Input: part model. Units: mm. Frame: model coordinates. A direction names the side the tool comes from. Round coordinates to 2 decimals unless told otherwise and drop trailing zeros. Loops run counter-clockwise (first coordinate to the right, second up) from the corner with the lowest first, then second, coordinate; pieces in that order, holes last. Notation, with made-up numbers: (80.25, -7) -> (119.25, -7) arc R6 cw to (119.25, 2) -> close; hole circle Ø8 at (27, -7). An arc over 180 degrees is marked (long way). One line per question, with ' | ' between items. Start each with the question number.
Q1. Access query for faces 4 (the face through (3, -15, 7.938)), 5 (the face through (-4.336, -19.524, 2.348)), 6 (the face through (-1, -22, 0)). Directions: +Z, -Z, +X, -X, +Y, -Y. A direction counts if a zero-diameter tool reaches every point of the face in a straight line with its end or side. Return the directions, or none.
Q2. Mould query, pull axis X, two halves, no side actions, for faces 1 (the face through (-1, -22, 12.7)), 2 (the face through (3, -15, 4.762)), 3 (the face through (47.69, 15.02, 6.26)). Classes: pulls with the +X half, pulls with the -X half, needs draft (parallel to the pull), parting line crosses it, or undercut.
Q3. Cut plane D-D on y = 28. Return loops of the section in (x, z).
Q4. Cut plane C-C on z = 3.25. Return loops of the section in (x, y), and give its area (3 significant figures).
Q5. Cut plane A-A on y = 0. Return loops of the section in (x, z), and give its area (3 significant figures).
Q6. Contact query for flat-ended pins moving along their axis: P1, Ø5, axis at x = 31, z = 8, coming from the +Y side; P2, Ø5, axis at y = 5.5, z = 8.5, coming from the +X side; P3, Ø1, axis at x = -32, z = 8, coming from the -Y side; P4, Ø12, axis at x = 3.5, y = -3, coming from the +Z side. Output: stop coordinate, or through.
Q7. Material intervals for L1, parallel to Y at x = 0, z = 9.65; L2, parallel to Y at x = 0, z = 5.75; L3, parallel to X at y = 18, z = 1, sorted ascending.
from build123d import *

# Parameters (mm, degrees)
F0_R     = 50
F0_R_2   = 20
F1_DEPTH = 12.7
F3_R     = 20
F3_R_2   = 15
F4_DEPTH = 1.5875


with BuildPart() as f1:
    # F0 (on Top) → F1 (new body)
    with BuildSketch(Plane.XY):
        Circle(F0_R)
        Circle(F0_R_2, mode=Mode.SUBTRACT)
    extrude(amount=F1_DEPTH)

    # F3 (on mid) → F4 (join, symmetric)
    with BuildSketch(Plane(origin=(0, 0, 6.35), x_dir=(1, 0, 0), z_dir=(0, 0, -1))):
        Circle(F3_R)
        Circle(F3_R_2, mode=Mode.SUBTRACT)
    extrude(amount=F4_DEPTH, both=True)


solid = f1.part
Results:
1) face 4: +Z | face 5: -Z | face 6: -Z, +X, -X, +Y, -Y
2) face 1: needs draft | face 2: undercut | face 3: parting line crosses it
3) outline: (-41.42, 0) -> (41.42, 0) -> (41.42, 12.7) -> (-41.42, 12.7) -> close
4) outline: circle Ø100 at (0, 0); hole circle Ø40 at (0, 0) | area: 6,600 mm^2
5) outline: (-50, 0) -> (-20, 0) -> (-20, 4.76) -> (-15, 4.76) -> (-15, 7.94) -> (-20, 7.94) -> (-20, 12.7) -> (-50, 12.7) -> close; (15, 4.76) -> (20, 4.76) -> (20, 0) -> (50, 0) -> (50, 12.7) -> (20, 12.7) -> (20, 7.94) -> (15, 7.94) -> close | area: 794 mm^2
6) P1: y = 41.08 | P2: x = 49.91 | P3: y = -38.83 | P4: through
7) L1: -50 to -20, 20 to 50 | L2: -50 to -15, 15 to 50 | L3: -46.65 to -8.72, 8.72 to 46.65
